Verification items for the finished model (mm, model axes). Give positions to 0.01 mm unless a question says otherwise; leave off trailing zeros. Loops run counter-clockwise (first coordinate to the right, second up) from the corner with the lowest first, then second, coordinate; pieces in that order, holes last. Notation, with made-up numbers: (-23, 5.5) - (11, 5.5) arc R29 ccw to (11, 38.5) - close; hole circle Ø3 at (-25, -26.75). An arc over 180 degrees is marked (long way). One line per item, written item: value. Start each with the question number.
1. Scan lines: L1, parallel to Z at x = -4, y = 4.1; L2, parallel to Z at x = -6.5, y = 4.25; L3, parallel to Z at x = 35, y = 2.8. Record each from-to range of solid material in increasing order. Write a range as [from, to].
2. Gauge pin test, flat end, axial feed: pin 1 (2 mm diameter, centred on x = -39.5, y = 1.5, fed in from +Z) (3 decimals). Record the tip position at first contact, or that the pin passes through.
3. Sectioned sample at B-B (z = 0). Record the cut outline in (x, y).
4. Sectioned sample at A-A (x = 0). Record the cut outline in (y, z), plus the area to 3 significant figures.
5. Mould release check, pull along Z, two halves, no side actions. Record for faces 1 (the cylindrical face through (7.493, 2.465, -0.33)), 2 (the flat face through (12, 0, 6)): pulls with the +Z half, pulls with the -Z half, needs draft (parallel to the pull), parting line crosses it, or undercut.
Autodesk Inventor part; units mm, degrees
ref_plane "YZ Plane" through (0, 0, 0) normal (1, 0, 0) x (0, 1, 0)
ref_plane "XZ Plane" through (0, 0, 0) normal (0, 1, 0) x (-1, 0, 0)
ref_plane "XY Plane" through (0, 0, 0) normal (0, 0, 1) x (1, 0, 0)
sketch "Sketch1" plane through (0, 0, 0) normal (0, 1, 0) x (-1, 0, 0)
  line L0 (0, 272.2446) -> (0, -272.2446) construction
  line L1 (50, 435.2374) -> (50, -435.2374)
  line L2 (-50, 435.2374) -> (-50, -435.2374)
  arc A0 (50, 435.2374) -> (-50, 435.2374) centre (0, 0) ccw
  arc A1 (-50, -435.2374) -> (50, -435.2374) centre (0, 0) ccw
  circle A2 centre (0, 0) radius 7.5
  dimension "d1" = 438.1
  dimension "d2" = 438.1
  dimension "d3" = 100
  dimension "d6" = 15
extrude "Extrusion1" add sketch "Sketch1" along normal blind 5
properties part number "rotorV1"
Results are:
1. L1: z = [-438.08, -6.34], [6.34, 438.08]
1. L2: z = [-438.05, -3.74], [3.74, 438.05]
1. L3: z = [-436.7, 436.7]
2. pin 1: stops at z = 436.405
3. outline: (-50, 0) - (-7.5, 0) - (-7.5, 5) - (-50, 5) - close; (7.5, 0) - (50, 0) - (50, 5) - (7.5, 5) - close
4. outline: (0, -438.1) - (5, -438.1) - (5, -7.5) - (0, -7.5) - close; (0, 7.5) - (5, 7.5) - (5, 438.1) - (0, 438.1) - close
4. area: 4,310 mm^2
5. face 1: undercut
5. face 2: needs draft
